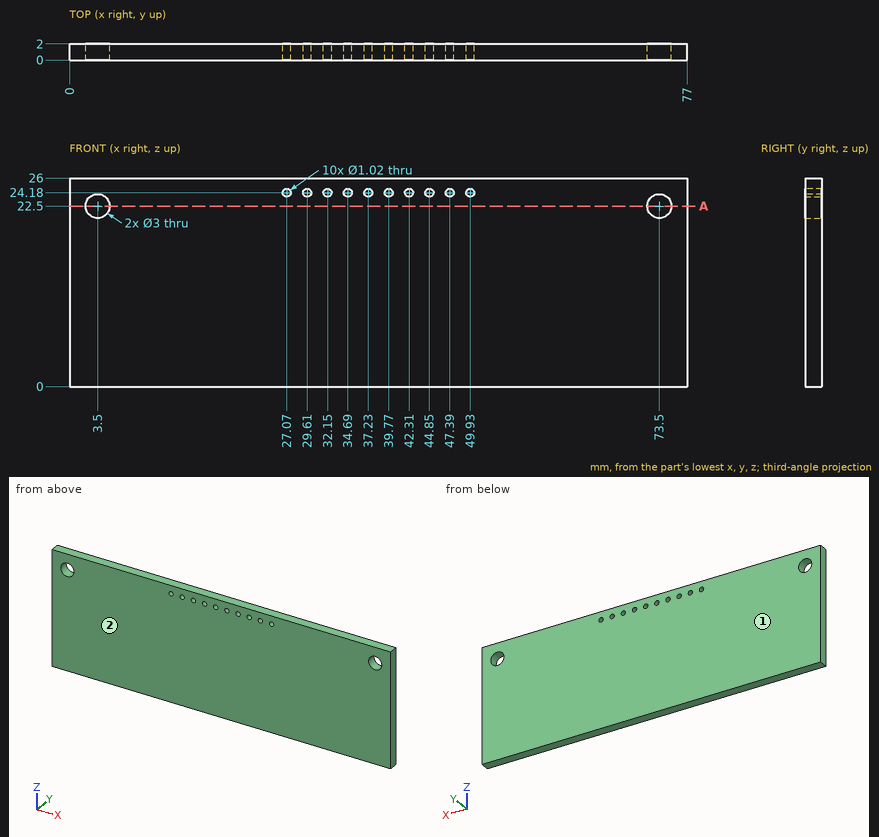
Source: three-view drawing plus pictorial views. Frame: mm from the lowest corner of the part. Round coordinates to 2 decimals unless told otherwise and drop trailing zeros. Write each loop counter-clockwise with the first axis right and the second up, starting at its lowest first coordinate (ties: lowest second). Pieces come first, ordered by that corner, then holes. Notation, with made-up numbers: (19.5, 0.5) -> (36.5, 0.5) arc R13 ccw to (36.5, 23.5) -> close; hole circle Ø2 at (9, -4). An arc over 180 degrees is marked (long way). Return JSON: item names as keys, results as strings.
Q1. Mould query, pull axis Y, two halves, no side actions, for the marked faces 1 and 2. Classes: +Y half, -Y half, draft (parallel to the pull), parting line (faces both ways), or undercut.
From the geometry:
{"face 1": "+Y half", "face 2": "-Y half"}
Q2. First-contact query: pin 1 Ø2.5 at (x, z) = (73.5, 22.5) entering from -Y. Flat tip, straight axial feed; report the tip coordinate or a pass-through.
From the geometry:
{"pin 1": "through"}
Q3. Section A-A on z = 22.5. Return the cut outline in (x, y).
From the geometry:
{"outline": "(0, 0) -> (2, 0) -> (2, 2) -> (0, 2) -> close; (5, 0) -> (72, 0) -> (72, 2) -> (5, 2) -> close; (75, 0) -> (77, 0) -> (77, 2) -> (75, 2) -> close"}
Q4. Ray query, line 1 (X direction, y = 0.9, z = 22.5); line 2 (X direction, y = 0.85, z = 23) (1 decimal); line 3 (Z direction, x = 73.5, y = 1.3). Return the intervals inside material, ascending.
From the geometry:
{"line 1": "0 to 2, 5 to 72, 75 to 77", "line 2": "0 to 2.1, 4.9 to 72.1, 74.9 to 77", "line 3": "0 to 21, 24 to 26"}
